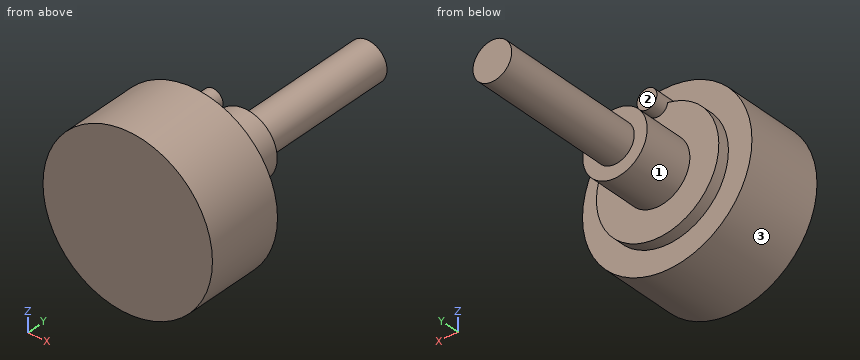
from build123d import *

# Parameters (mm, degrees)
SKETCH1_R           = 13.15
BOSS_EXTRUDE1_DEPTH = 12.2
SKETCH2_R           = 9.5
BOSS_EXTRUDE2_DEPTH = 1.8
SKETCH3_R           = 5
BOSS_EXTRUDE3_DEPTH = 8
SKETCH4_R           = 3
BOSS_EXTRUDE4_DEPTH = 23
SKETCH5_R           = 1.55
BOSS_EXTRUDE5_DEPTH = 3.8


with BuildPart() as part:
    # Sketch1 → Boss-Extrude1 (new body)
    with BuildSketch(Plane(origin=(0, 0, 0), x_dir=(1, 0, 0), z_dir=(0, 1, 0))):
        Circle(SKETCH1_R)
    extrude(amount=BOSS_EXTRUDE1_DEPTH)

    # Sketch2 → Boss-Extrude2 (add)
    with BuildSketch(Plane(origin=(0, 12.2, 0), x_dir=(1, 0, 0), z_dir=(0, 1, 0))):
        Circle(SKETCH2_R)
    extrude(amount=BOSS_EXTRUDE2_DEPTH)

    # Sketch3 → Boss-Extrude3 (add)
    with BuildSketch(Plane(origin=(0, 14, 0), x_dir=(1, 0, 0), z_dir=(0, 1, 0))):
        Circle(SKETCH3_R)
    extrude(amount=BOSS_EXTRUDE3_DEPTH)

    # Sketch4 → Boss-Extrude4 (add)
    with BuildSketch(Plane(origin=(0, 22, 0), x_dir=(1, 0, 0), z_dir=(0, 1, 0))):
        Circle(SKETCH4_R)
    extrude(amount=BOSS_EXTRUDE4_DEPTH)

    # Sketch5 → Boss-Extrude5 (add)
    with BuildSketch(Plane(origin=(0, 12.2, 0), x_dir=(1, 0, 0), z_dir=(0, 1, 0))):
        with Locations((0, -9.5)):
            Circle(SKETCH5_R)
    extrude(amount=BOSS_EXTRUDE5_DEPTH)


solid = part.part
The model under review builds one solid part; all positions refer to its coordinate system, in mm. Face numbers are marked on the shaded views. A direction names the side the tool comes from. Give positions to 0.01 mm unless a question says otherwise; leave off trailing zeros. Order: outer loops, then holes, each group sorted by start corner. A loop starts at its lowest first (then second) coordinate and runs counter-clockwise, first axis right, second up. Notation, with made-up numbers: (55, 53) -> (90, 53) arc R16 cw to (90, 71) -> close; hole circle Ø10 at (10, -21). An arc over 180 degrees is marked (long way). Write item = value, one per line. Start each with the question number.
(1) Tool access review of the marked faces 1, 2 and 3: name each direction out of +Z, -Z, +X, -X, +Y, -Y from which nothing blocks a thin tool from reaching the whole face with its end or side.
(2) For pin 1 Ø0.9 at (x, z) = (0.5, 10) entering from +Y; pin 2 Ø6 at (y, z) = (24.5, -1.5) entering from +X; pin 3 Ø6 at (y, z) = (29.5, -2) entering from +X, all flat-tipped, find the tip position at first contact; note any pin that passes through.
(3) Take a section at C-C (y = 10.5). Write out the cut boundary in (x, z).
(4) Take a section at B-B (x = -6.25). Write out the cut boundary in (y, z).
(5) Take a section at A-A (z = 0). Write out the cut boundary in (x, y).
(6) For L1, parallel to Y at x = -4.5, z = -7.5; L2, parallel to Y at x = 9.75, z = -1.25; L3, parallel to X at y = 11, z = -8, list the stretches that pass through material, from the lowest coordinate up. Write a range as from..to.
(7) Take a section at D-D (x = 0). Write out the cut boundary in (y, z), plus the area to 3 significant figures.
Returned:
q1.face_1 = +Y
q1.face_2 = +Z, +X, -X, +Y
q1.face_3 = +Y, -Y
q2.pin_1 = 16
q2.pin_2 = 5
q2.pin_3 = 3
q3.outline = circle Ø26.3 at (0, 0)
q4.outline = (0, -11.57) -> (12.2, -11.57) -> (12.2, -7.15) -> (14, -7.15) -> (14, 7.15) -> (12.2, 7.15) -> (12.2, 11.57) -> (0, 11.57) -> close
q5.outline = (-13.15, 0) -> (13.15, 0) -> (13.15, 12.2) -> (9.5, 12.2) -> (9.5, 14) -> (5, 14) -> (5, 22) -> (3, 22) -> (3, 45) -> (-3, 45) -> (-3, 22) -> (-5, 22) -> (-5, 14) -> (-9.5, 14) -> (-9.5, 12.2) -> (-13.15, 12.2) -> close
q6.L1 = 0..14
q6.L2 = 0..12.2
q6.L3 = -10.44..10.44
q7.outline = (0, -13.15) -> (12.2, -13.15) -> (12.2, -9.5) -> (14, -9.5) -> (14, -5) -> (22, -5) -> (22, -3) -> (45, -3) -> (45, 3) -> (22, 3) -> (22, 5) -> (14, 5) -> (14, 7.95) -> (16, 7.95) -> (16, 11.05) -> (12.2, 11.05) -> (12.2, 13.15) -> (0, 13.15) -> close
q7.area = 582 mm²
